Build history of the part. All positions in model axes, mm. A direction names the side the tool comes from. Round coordinates to 2 decimals unless told otherwise and drop trailing zeros. Write each loop counter-clockwise with the first axis right and the second up, starting at its lowest first coordinate (ties: lowest second). Pieces come first, ordered by that corner, then holes. Notation, with made-up numbers: (57.5, 78) -> (88.5, 78) arc R26 ccw to (88.5, 105) -> close; hole circle Ø3 at (-14.75, 28.25). An arc over 180 degrees is marked (long way). Return JSON: item names as keys, results as strings.
from build123d import *

# Parameters (mm, degrees)
ESQUISSE1_R        = 3.25
ESQUISSE1_R_2      = 3.5
BOSS_EXTRU_1_DEPTH = 10
CONG_1_R           = 6
CONG_2_R           = 8
CONG_3_R           = 7
CONG_4_R           = 2


with BuildPart() as part:
    # Esquisse1 → Boss.-Extru.1 (new body)
    with BuildSketch(Plane.XY):
        Polygon((24, 110), (24, 36), (0, 36), (0, 30), (14, 30), (16.721324328, 16), (34, 16), (34, 110), align=None)
        with Locations((29, 104)):
            Circle(ESQUISSE1_R, mode=Mode.SUBTRACT)
        with Locations((22, 23)):
            Circle(ESQUISSE1_R_2, mode=Mode.SUBTRACT)
        with Locations((29, 70)):
            Circle(ESQUISSE1_R, mode=Mode.SUBTRACT)
    boss_extru_1 = extrude(amount=BOSS_EXTRU_1_DEPTH)

    # Symétrie2: Boss.-Extru.1 across plane
    add(boss_extru_1.mirror(Plane(origin=(0, 36, 10), x_dir=(0, 0, 1), z_dir=(1, 0, 0))))

    # Congé1
    cong_1_edges = [part.edges().sort_by_distance(p)[0] for p in [
        (16.721324328, 16, 5),
        (14, 30, 5),
        (-14, 30, 5),
        (-16.721324328, 16, 5),
    ]]
    fillet(cong_1_edges, radius=CONG_1_R)

    # Congé2
    cong_2_edges = [part.edges().sort_by_distance(p)[0] for p in [
        (34, 16, 5),
        (-34, 16, 5),
    ]]
    fillet(cong_2_edges, radius=CONG_2_R)

    # Congé3
    cong_3_edges = [part.edges().sort_by_distance(p)[0] for p in [
        (34, 110, 5),
        (-34, 110, 5),
    ]]
    fillet(cong_3_edges, radius=CONG_3_R)

    # Congé4
    cong_4_edges = [part.edges().sort_by_distance(p)[0] for p in [
        (24, 36, 5),
        (-24, 36, 5),
    ]]
    fillet(cong_4_edges, radius=CONG_4_R)


solid = part.part
Q1. Saw through at A-A on y = 44. List the corners of the cut face in (x, z).
Verdict:
{"outline": "(-34, 0) -> (-24, 0) -> (-24, 10) -> (-34, 10) -> close; (24, 0) -> (34, 0) -> (34, 10) -> (24, 10) -> close"}
Q2. Wall check: L1, parallel to X at y = 74.5, z = 7.5; L2, parallel to Y at x = 22, z = 6.5; L3, parallel to X at y = 68.5, z = 7. Give the ranges that are in metal, low to high.
Verdict:
{"L1": "x = -34 to -24, 24 to 34", "L2": "y = 16 to 19.5, 26.5 to 36", "L3": "x = -34 to -31.88, -26.12 to -24, 24 to 26.12, 31.88 to 34"}
Q3. Saw through at C-C on x = 30.5. List the corners of the cut face in (y, z), then the cut area to 3 significant figures.
Verdict:
{"outline": "(17.39, 0) -> (67.12, 0) -> (67.12, 10) -> (17.39, 10) -> close; (72.88, 0) -> (101.12, 0) -> (101.12, 10) -> (72.88, 10) -> close; (106.88, 0) -> (109.06, 0) -> (109.06, 10) -> (106.88, 10) -> close", "area": "801 mm²"}
Q4. Saw through at B-B on y = 70. List the corners of the cut face in (x, z), then the cut area to 3 significant figures.
Verdict:
{"outline": "(-34, 0) -> (-32.25, 0) -> (-32.25, 10) -> (-34, 10) -> close; (-25.75, 0) -> (-24, 0) -> (-24, 10) -> (-25.75, 10) -> close; (24, 0) -> (25.75, 0) -> (25.75, 10) -> (24, 10) -> close; (32.25, 0) -> (34, 0) -> (34, 10) -> (32.25, 10) -> close", "area": "70.0 mm²"}
Q5. Two-plate mould, pull along X, no slides. Class faces 4 (the cylindrical face through (31.594, 18.281, 5.07)), 5 (the cylindrical face through (12.826, 28.666, 5.07)), 6 (the flat face through (24, 16, 5)), 7 (the flat face through (-34, 63, 5)): +X half, -X half, draft (parallel to the pull), parting line (faces both ways), or undercut.
Verdict:
{"face 4": "+X half", "face 5": "undercut", "face 6": "draft", "face 7": "-X half"}
Q6. 3-axis set-ups, long thin cutter, end or side, ignore diameter. For faces 1 (the flat face through (0, 36, 5)), 2 (the cylindrical face through (30.5, 101.117, 4.93)), 3 (the cylindrical face through (17.806, 17.407, 5.07)): which of +Z, -Z, +X, -X, +Y, -Y reach the whole face in a straight line?
Verdict:
{"face 1": "+Z, -Z, +Y", "face 2": "+Z, -Z", "face 3": "+Z, -Z, -Y"}
Q7. Pin check, flat tips, straight feed: pin 1 Ø8 at (x, y) = (-22, 23) entering from +Z; pin 2 Ø5 at (x, y) = (29, 104) entering from -Z; pin 3 Ø6 at (x, z) = (2, 5.5) entering from -Y. Stop position of each tip, or through.
Verdict:
{"pin 1": "stops at z = 10", "pin 2": "passes through", "pin 3": "stops at y = 30"}
Q8. Saw through at D-D on z = 1. List the corners of the cut face in (x, y).
Verdict:
{"outline": "(-34, 24) arc R8 ccw to (-26, 16) -> (-21.67, 16) arc R6 ccw to (-15.78, 20.86) -> (-14.94, 25.14) arc R6 cw to (-9.05, 30) -> (9.05, 30) arc R6 cw to (14.94, 25.14) -> (15.78, 20.86) arc R6 ccw to (21.67, 16) -> (26, 16) arc R8 ccw to (34, 24) -> (34, 103) arc R7 ccw to (27, 110) -> (24, 110) -> (24, 38) arc R2 cw to (22, 36) -> (-22, 36) arc R2 cw to (-24, 38) -> (-24, 110) -> (-27, 110) arc R7 ccw to (-34, 103) -> close; hole circle Ø6.5 at (-29, 70); hole circle Ø6.5 at (-29, 104); hole circle Ø7 at (-22, 23); hole circle Ø7 at (22, 23); hole circle Ø6.5 at (29, 70); hole circle Ø6.5 at (29, 104)"}
